from build123d import *

# Parameters (mm, degrees)
SKETCH_1_R               = 10
SKETCH_1_R_2             = 6.05
EXTRUDE_1_DEPTH          = 2
SKETCH_2_R               = 1.65
CUT_EXTRUDE_1_DEPTH      = 2
PATTERN_CIRCULAR_1_COUNT = 4
SKETCH_3_R               = 11
SKETCH_3_R_2             = 10
EXTRUDE_2_DEPTH          = 1.5
SKETCH_4_R               = 3
CUT_EXTRUDE_2_DEPTH      = 2.5
PATTERN_CIRCULAR_2_COUNT = 4


with BuildPart() as part:
    # 草图1 → 凸台-拉伸1 (new body)
    with BuildSketch(Plane(origin=(0, 0, 0), x_dir=(1, 0, 0), z_dir=(0, 1, 0))):
        with Locations(Location((0, 0, 0), (0, 0, 270))):
            Circle(SKETCH_1_R)
        with Locations(Location((0, 0, 0), (0, 0, 270))):
            Circle(SKETCH_1_R_2, mode=Mode.SUBTRACT)
    extrude(amount=EXTRUDE_1_DEPTH)

    # 草图2 → 切除-拉伸1 (cut)
    with BuildSketch(Plane(origin=(0, 2, 0), x_dir=(1, 0, 0), z_dir=(0, 1, 0))):
        with Locations((-6.5, 0)):
            Circle(SKETCH_2_R)
    cut_extrude_1 = extrude(amount=-CUT_EXTRUDE_1_DEPTH, mode=Mode.SUBTRACT)

    # 阵列(圆周)1: 切除-拉伸1 ×4 about axis
    pattern_circular_1_axis = Axis((0, 0, 0), (0, 1, 0))
    for i in range(1, PATTERN_CIRCULAR_1_COUNT):
        add(cut_extrude_1.rotate(pattern_circular_1_axis, i * 360 / PATTERN_CIRCULAR_1_COUNT), mode=Mode.SUBTRACT)

    # 草图3 → 凸台-拉伸2 (add)
    # profile 1 of 2: a face of its own
    with BuildSketch(Plane(origin=(0, 2, 0), x_dir=(1, 0, 0), z_dir=(0, 1, 0))):
        with Locations(Location((0, 0, 0), (0, 0, 270))):
            Circle(SKETCH_3_R)
        with Locations(Location((0, 0, 0), (0, 0, 270))):
            Circle(SKETCH_3_R_2, mode=Mode.SUBTRACT)
    # profile 2 of 2: a face of its own
    with BuildSketch(Plane(origin=(0, 2, 0), x_dir=(1, 0, 0), z_dir=(0, 1, 0))):
        with Locations(Location((0, 0, 0), (0, 0, 270))):
            Circle(SKETCH_3_R_2)
        with BuildLine():
            ThreePointArc((5.856153846, -1.519197857), (4.277996026, -4.277996026), (1.519197857, -5.856153846))
            ThreePointArc((1.519197857, -5.856153846), (0, -8.15), (-1.519197857, -5.856153846))
            ThreePointArc((-1.519197857, -5.856153846), (-4.277996026, -4.277996026), (-5.856153846, -1.519197857))
            ThreePointArc((-5.856153846, -1.519197857), (-8.15, 0), (-5.856153846, 1.519197857))
            ThreePointArc((-5.856153846, 1.519197857), (-4.277996026, 4.277996026), (-1.519197857, 5.856153846))
            ThreePointArc((-1.519197857, 5.856153846), (0, 8.15), (1.519197857, 5.856153846))
            ThreePointArc((1.519197857, 5.856153846), (4.277996026, 4.277996026), (5.856153846, 1.519197857))
            ThreePointArc((5.856153846, 1.519197857), (8.15, 0), (5.856153846, -1.519197857))
        make_face(mode=Mode.SUBTRACT)
    extrude(amount=EXTRUDE_2_DEPTH)

    # 草图4 → 切除-拉伸2 (cut)
    with BuildSketch(Plane(origin=(0, 3.5, 0), x_dir=(1, 0, 0), z_dir=(0, 1, 0))):
        with Locations((-6.5, 0)):
            Circle(SKETCH_4_R)
    cut_extrude_2 = extrude(amount=-CUT_EXTRUDE_2_DEPTH, mode=Mode.SUBTRACT)

    # 阵列(圆周)2: 切除-拉伸2 ×4 about axis
    pattern_circular_2_axis = Axis((0, 0, 0), (0, 1, 0))
    for i in range(1, PATTERN_CIRCULAR_2_COUNT):
        add(cut_extrude_2.rotate(pattern_circular_2_axis, i * 360 / PATTERN_CIRCULAR_2_COUNT), mode=Mode.SUBTRACT)


solid = part.part
Read the model definition and answer for the solid it produces. Units are mm, in the model's axes. A direction names the side the tool comes from. Give positions to 0.01 mm unless a question says otherwise; leave off trailing zeros. Loops run counter-clockwise (first coordinate to the right, second up) from the corner with the lowest first, then second, coordinate; pieces in that order, holes last. Notation, with made-up numbers: (-4, -20.75) -> (53, -20.75) arc R28 cw to (53, 0.25) -> close; hole circle Ø5 at (-9.5, 22.25). An arc over 180 degrees is marked (long way). Use a Markdown table: item, result.
Q1. A tool of negligible diameter and unlimited length cuts with its end or side. For faces 1 (the face through (-10, 2, 2)), 2 (the face through (-0.05, 0.51, 8.15)), 3 (the face through (-0.1, 2.3, 9.5)), from which of +Z, -Z, +X, -X, +Y, -Y can it reach the whole face along a straight path? Write none if from no direction.
Solved:
| item | result |
|---|---|
| face 1 | -Y |
| face 2 | +Y, -Y |
| face 3 | +Y |
Q2. Determine the mould class of faces 4 (the face through (-9.76, 0.99, -2.17)), 5 (the face through (-9.5, 2.3, -0.1)), 6 (the face through (-5, 3.5, 5)) for opening direction Z: pulls with the +Z half, pulls with the -Z half, needs draft (parallel to the pull), parting line crosses it, or undercut.
Solved:
| item | result |
|---|---|
| face 4 | parting line crosses it |
| face 5 | undercut |
| face 6 | needs draft |
Q3. Each of these flat-tipped pins is pushed along its axis until it touches: pin 1 (1.2 mm diameter, centred on x = 1.5, z = 7, fed in from +Y); pin 2 (2 mm diameter, centred on y = 1.5, z = -6, fed in from -X); pin 3 (2 mm diameter, centred on x = 2.5, y = 2.5, fed in from -Z). Where does it stop, or does it pass through?
Solved:
| item | result |
|---|---|
| pin 1 | stops at y = 1 |
| pin 2 | stops at x = -9.73 |
| pin 3 | stops at z = -10.9 |
Q4. Section D-D, the plane y = 0.45 is taken. Determine the outline of the cut face in (x, z).
Solved:
| item | result |
|---|---|
| outline | circle Ø20 at (0, 0); hole (-5.86, -1.52) arc R6.05 ccw to (-1.52, -5.86) arc R1.65 ccw (long way) to (1.52, -5.86) arc R6.05 ccw to (5.86, -1.52) arc R1.65 ccw (long way) to (5.86, 1.52) arc R6.05 ccw to (1.52, 5.86) arc R1.65 ccw (long way) to (-1.52, 5.86) arc R6.05 ccw to (-5.86, 1.52) arc R1.65 ccw (long way) to start |
Q5. Section A-A, the plane z = 0 is taken. Determine the outline of the cut face in (x, y), then the cut area to 3 significant figures.
Solved:
| item | result |
|---|---|
| outline | (-11, 2) -> (-10, 2) -> (-10, 0) -> (-8.15, 0) -> (-8.15, 1) -> (-9.5, 1) -> (-9.5, 3.5) -> (-11, 3.5) -> close; (8.15, 0) -> (10, 0) -> (10, 2) -> (11, 2) -> (11, 3.5) -> (9.5, 3.5) -> (9.5, 1) -> (8.15, 1) -> close |
| area | 9.20 mm^2 |
Q6. Section C-C, the plane x = 6.5 is taken. Determine the outline of the cut face in (y, z).
Solved:
| item | result |
|---|---|
| outline | (0, -7.6) -> (2, -7.6) -> (2, -8.87) -> (3.5, -8.87) -> (3.5, -3) -> (1, -3) -> (1, -1.65) -> (0, -1.65) -> close; (0, 1.65) -> (1, 1.65) -> (1, 3) -> (3.5, 3) -> (3.5, 8.87) -> (2, 8.87) -> (2, 7.6) -> (0, 7.6) -> close |
Q7. Section B-B, the plane y = 2.5 is taken. Determine the outline of the cut face in (x, z), then the cut area to 3 significant figures.
Solved:
| item | result |
|---|---|
| outline | circle Ø22 at (0, 0); hole (-5.37, -2.78) arc R6.05 ccw to (-2.78, -5.37) arc R3 ccw (long way) to (2.78, -5.37) arc R6.05 ccw to (5.37, -2.78) arc R3 ccw (long way) to (5.37, 2.78) arc R6.05 ccw to (2.78, 5.37) arc R3 ccw (long way) to (-2.78, 5.37) arc R6.05 ccw to (-5.37, 2.78) arc R3 ccw (long way) to start |
| area | 192 mm^2 |
Q8. Find the intervals of material crossed by line 1 along X through (y, z) = (3, 0); line 2 along Z through (x, y) = (-9.25, 1.85); line 3 along X through (y, z) = (0.5, 6.5), in increasing order.
Solved:
| item | result |
|---|---|
| line 1 | x = -11 to -9.5, 9.5 to 11 |
| line 2 | z = -3.8 to -1.2, 1.2 to 3.8 |
| line 3 | x = -7.6 to -1.65, 1.65 to 7.6 |
